Model file for the job. Use its own axes, mm. A direction names the side the tool comes from. Give positions to 0.01 mm unless a question says otherwise; leave off trailing zeros. Order: outer loops, then holes, each group sorted by start corner. A loop starts at its lowest first (then second) coordinate and runs counter-clockwise, first axis right, second up. Notation, with made-up numbers: (55, -15.75) -> (99, -15.75) arc R15 cw to (99, 8.25) -> close; hole circle Ø10 at (66, 44). An arc over 180 degrees is marked (long way). Answer in a Markdown table with one row per item. Add a question column.
from build123d import *

# Parameters (mm, degrees)
SKETCH1_W           = 200
SKETCH1_H           = 20
SKETCH1_W_2         = 7.6
SKETCH1_H_2         = 5.1
BOSS_EXTRUDE1_DEPTH = 6
SKETCH2_W           = 20.1
SKETCH2_H           = 20
CUT_EXTRUDE1_DEPTH  = 3
FILLET1_R           = 1


with BuildPart() as part:
    # Sketch1 → Boss-Extrude1 (new body)
    with BuildSketch(Plane(origin=(0, 0, 0), x_dir=(1, 0, 0), z_dir=(0, 1, 0))):
        Rectangle(SKETCH1_W, SKETCH1_H)
        with Locations((-90, 0)):
            Rectangle(SKETCH1_W_2, SKETCH1_H_2, mode=Mode.SUBTRACT)
        with Locations((90, 0)):
            Rectangle(SKETCH1_W_2, SKETCH1_H_2, mode=Mode.SUBTRACT)
    extrude(amount=BOSS_EXTRUDE1_DEPTH)

    # Sketch2 → Cut-Extrude1 (cut)
    with BuildSketch(Plane(origin=(0, 6, 0), x_dir=(1, 0, 0), z_dir=(0, 1, 0))):
        with Locations((-89.95, 0)):
            Rectangle(SKETCH2_W, SKETCH2_H)
        with Locations((89.95, 0)):
            Rectangle(SKETCH2_W, SKETCH2_H)
    extrude(amount=-CUT_EXTRUDE1_DEPTH, mode=Mode.SUBTRACT)

    # Fillet1
    fillet1_edges = [part.edges().sort_by_distance(p)[0] for p in [
        (-100, 3, 0),
        (-89.95, 3, -10),
        (-89.95, 3, 10),
        (-79.9, 6, 0),
        (100, 3, 0),
        (89.95, 3, 10),
        (89.95, 3, -10),
        (79.9, 6, 0),
    ]]
    fillet(fillet1_edges, radius=FILLET1_R)


solid = part.part
Item 1: Saw through at D-D on z = 7.25. List the corners of the cut face in (x, y), plus the area to 3 significant figures.
Item 2: Wall check: line 1 (X direction, y = 0.3, z = -0.75); line 2 (X direction, y = 2.9, z = -0.25); line 3 (X direction, y = 3.3, z = 7.5). Give the ranges that are in metal, low to high.
Item 3: Saw through at A-A on z = -0.75. List the corners of the cut face in (x, y), plus the area to 3 significant figures.
Item 4: Which spindle directions (+Z, -Z, +X, -X, +Y, -Y) get a long thin tool onto all of the face, cutting with end or side? Do faces 1 (the flat face through (89, 3, -4)), 2 (the flat face through (-90, 3, -4)), 3 (the flat face through (-1, 3, -10)). Say none if no direction does.
Item 5: Saw through at C-C on y = 1.05. List the corners of the cut face in (x, z), plus the area to 3 significant figures.
Item 6: Saw through at B-B on x = 88.5. List the corners of the cut face in (y, z), plus the area to 3 significant figures.
Item 7: Pin check, flat tips, straight feed: pin 1 Ø1.5 at (y, z) = (3, -3) entering from -X; pin 2 Ø1.5 at (y, z) = (3.5, -0.5) entering from -X; pin 3 Ø1.5 at (y, z) = (4.5, -1.5) entering from +X. Stop position of each tip, or through.
Evaluation:
| question | item | result |
|---|---|---|
| 1 | outline | (-100, 0) -> (100, 0) -> (100, 2) arc R1 ccw to (99, 3) -> (79.9, 3) -> (79.9, 5) arc R1 ccw to (78.9, 6) -> (-78.9, 6) arc R1 ccw to (-79.9, 5) -> (-79.9, 3) -> (-99, 3) arc R1 ccw to (-100, 2) -> close |
| 1 | area | 1,080 mm2 |
| 2 | line 1 | x = -100 to -93.8, -86.2 to 86.2, 93.8 to 100 |
| 2 | line 2 | x = -99.44 to -93.8, -86.2 to 86.2, 93.8 to 99.44 |
| 2 | line 3 | x = -79.9 to 79.9 |
| 3 | outline | (-100, 0) -> (-93.8, 0) -> (-93.8, 3) -> (-99, 3) arc R1 ccw to (-100, 2) -> close; (-86.2, 0) -> (86.2, 0) -> (86.2, 3) -> (79.9, 3) -> (79.9, 5) arc R1 ccw to (78.9, 6) -> (-78.9, 6) arc R1 ccw to (-79.9, 5) -> (-79.9, 3) -> (-86.2, 3) -> close; (93.8, 0) -> (100, 0) -> (100, 2) arc R1 ccw to (99, 3) -> (93.8, 3) -> close |
| 3 | area | 1,030 mm2 |
| 4 | face 1 | +Z, -Z, +X, +Y |
| 4 | face 2 | +Z, -Z, -X, +Y |
| 4 | face 3 | -Z, +X, -X, +Y, -Y |
| 5 | outline | (-100, -10) -> (100, -10) -> (100, 10) -> (-100, 10) -> close; hole (-93.8, -2.55) -> (-86.2, -2.55) -> (-86.2, 2.55) -> (-93.8, 2.55) -> close; hole (86.2, -2.55) -> (93.8, -2.55) -> (93.8, 2.55) -> (86.2, 2.55) -> close |
| 5 | area | 3,920 mm2 |
| 6 | outline | (0, -10) -> (2, -10) arc R1 ccw to (3, -9) -> (3, -2.55) -> (0, -2.55) -> close; (0, 2.55) -> (3, 2.55) -> (3, 9) arc R1 ccw to (2, 10) -> (0, 10) -> close |
| 6 | area | 44.3 mm2 |
| 7 | pin 1 | stops at x = -99.97 |
| 7 | pin 2 | stops at x = -99.66 |
| 7 | pin 3 | stops at x = 79.9 |
